Autodesk Fusion 360 part; units mm, degrees
sketch "Sketch1" plane through (0, 0, 0) normal (0, 0, 1) x (1, 0, 0)
  circle A0 centre (0, 0) radius 3.5
  dimension "d1" = 7
extrude "Extrude1" add sketch "Sketch1" along normal blind 2
sketch "Sketch2" plane through (0, 0, 2) normal (0, 0, 1) x (-1, 0, 0)
  circle A0 centre (0, 0) radius 3.5
  line L0 (-1, 3) -> (1, 3)
  line L1 (1, -3) -> (-1, -3)
  line L2 (-3, -1) -> (-3, 1)
  line L3 (3, 1) -> (3, -1)
  line L4 (1, 3) -> (1, 1)
  line L5 (1, -1) -> (1, -3)
  line L6 (3, -1) -> (1, -1)
  line L7 (-1, -1) -> (-3, -1)
  line L8 (-1, -3) -> (-1, -1)
  line L9 (-1, 1) -> (-1, 3)
  line L10 (-3, 1) -> (-1, 1)
  line L11 (1, 1) -> (3, 1)
  dimension "d4" = 2
  dimension "d5" = 6
  dimension "d6" = 6
  dimension "d7" = 2
extrude "Extrude2" add sketch "Sketch2" along normal blind 10 contours L0 L1 L2 L3 L4 L5 L6 L7 L8 L9 L10 L11
sketch "Sketch3" plane through (0, 0, 0) normal (0, 0, 1) x (1, 0, 0)
  line L0 (1, 3) -> (-1, 3)
  line L1 (-1, -3) -> (1, -3)
  line L2 (3, 1) -> (3, -1)
  line L3 (-3, -1) -> (-3, 1)
  line L4 (-1, 3) -> (-1, 1)
  line L5 (-1, -1) -> (-1, -3)
  line L6 (3, -1) -> (1, -1)
  line L7 (-1, -1) -> (-3, -1)
  line L8 (1, -3) -> (1, -1)
  line L9 (1, 1) -> (1, 3)
  line L10 (-3, 1) -> (-1, 1)
  line L11 (1, 1) -> (3, 1)
  dimension "d10" = 2
  dimension "d11" = 6
  dimension "d12" = 6
  dimension "d13" = 2
extrude "Extrude3" add sketch "Sketch3" against normal blind 45
CAD build for the part. Positions are in the model's coordinates, mm. A direction names the side the tool comes from. Coordinates: 2 decimals unless noted, no trailing zeros. Loops run counter-clockwise (first coordinate to the right, second up) from the corner with the lowest first, then second, coordinate; pieces in that order, holes last. Notation, with made-up numbers: (61.25, 17) - (107.25, 17) arc R29 cw to (107.25, 37) - close; hole circle Ø7 at (63, 75). An arc over 180 degrees is marked (long way). Return JSON: item names as keys, results as strings.
1. Probe L1, parallel to Y at x = -0.75, z = -36; L2, parallel to Y at x = 2.25, z = -6.5. List the from-to ranges inside material, lowest first. Write a range as from..to.
Result:
{"L1": "y = -3..3", "L2": "y = -1..1"}
2. Drop flat-ended pins along their axis: pin 1 (1.6 mm diameter, centred on x = 2, z = -33, fed in from -Y); pin 2 (1.6 mm diameter, centred on y = -0.5, z = 8, fed in from -X); pin 3 (1.6 mm diameter, centred on x = -0.5, z = -20, fed in from +Y). Give the stop position or say it passes through.
Result:
{"pin 1": "stops at y = -1", "pin 2": "stops at x = -3", "pin 3": "stops at y = 3"}
3. Band-saw the part on B-B (z = -5). Give the cut face in (x, y).
Result:
{"outline": "(-3, -1) - (-1, -1) - (-1, -3) - (1, -3) - (1, -1) - (3, -1) - (3, 1) - (1, 1) - (1, 3) - (-1, 3) - (-1, 1) - (-3, 1) - close"}
4. 3-axis set-ups, long thin cutter, end or side, ignore diameter. For faces 1 (the flat face through (2, -1, 7)), 2 (the flat face through (3, 0, 7)), 3 (the flat face through (-1, -2, 7)), 4 (the flat face through (1, -2, -22)): which of +Z, -Z, +X, -X, +Y, -Y reach the whole face in a straight line?
Result:
{"face 1": "+Z, +X, -Y", "face 2": "+Z, +X, +Y, -Y", "face 3": "+Z, -X, -Y", "face 4": "-Z, +X, -Y"}
